from build123d import *


with BuildPart() as f1:
    # F0 (on Front) → F1 (revolve)
    with BuildSketch(Plane.XZ):
        with BuildLine():
            Line((0, 1.241046), (0, 2.482092))
            Line((0, 2.482092), (-22.902938, 2.482092))
            Line((-22.902938, 2.482092), (-22.902938, 0))
            Line((-22.902938, 0), (-24.024541, 0))
            Line((-24.024541, 0), (-30.056966, 73.394649))
            ThreePointArc((-30.056966, 73.394649), (-30.761444, 73.644653), (-30.481581, 72.951496))
            Line((-30.481581, 72.951496), (-24.376155, -1.331323))
            Line((-24.376155, -1.331323), (-22.775946, -1.199799))
            Line((-22.775946, -1.199799), (-21.772536, 1.241046))
            Line((-21.772536, 1.241046), (0, 1.241046))
        make_face()
    revolve(axis=Axis((0, 0, 1.861569), (0, 0, 1)))


solid = f1.part
Input: part model. Units: mm. Frame: model coordinates. A direction names the side the tool comes from. Coordinates: 2 decimals unless noted, no trailing zeros. Loops run counter-clockwise (first coordinate to the right, second up) from the corner with the lowest first, then second, coordinate; pieces in that order, holes last.
(1) Section D-D on z = 56. Return the cut outline in (x, y).
(2) First-contact query: pin 1 Ø12 at (x, z) = (4.5, 17) entering from -Y; pin 2 Ø8 at (x, z) = (24.5, 41) entering from +Y; pin 3 Ø12 at (y, z) = (10, 20.5) entering from +X. Flat tips, straight axial feed; report the tip coordinate or a pass-through.
(3) Pull-direction query (Y, two-part tool) for faces 3 (the face through (5.937, 26.735, 35.29)), 4 (the face through (5.87, 26.44, 37.21)), 5 (the face through (0, 0, 2.482)); classes: released by +Y, released by -Y, zero draft, split by the parting line, or undercut.
(4) Set-up query: faces 1 (the face through (19.5, 12.3, 0)), 2 (the face through (0, 0, 1.241)). Return all of +Z, -Z, +X, -X, +Y, -Y with unobstructed straight access to the full face (end or side cutting, diameter ignored); none if empty.
(5) Section A-A on y = 0. Return the cut outline in (x, z).
(6) Material intervals for probe 1 along Z at (x, y) = (-11.5, -17); probe 2 along X at (y, z) = (-17.5, 7); probe 3 along X at (y, z) = (1.5, 56), sorted ascending.
(7) Section C-C on z = 29. Return the cut outline in (x, y).
Data:
1. outline: circle Ø58.18 at (0, 0); hole circle Ø57.25 at (0, 0)
2. pin 1: stops at y = -26.27
2. pin 2: stops at y = 18.89
2. pin 3: stops at x = 25.98
3. face 3: split by the parting line
3. face 4: undercut
3. face 5: undercut
4. face 1: +Z
4. face 2: -Z
5. outline: (-30.48, 72.95) - (-24.38, -1.33) - (-22.78, -1.2) - (-21.77, 1.24) - (21.77, 1.24) - (22.78, -1.2) - (24.38, -1.33) - (30.48, 72.95) arc R0.41 ccw (long way) to (30.06, 73.39) - (24.02, 0) - (22.9, 0) - (22.9, 2.48) - (-22.9, 2.48) - (-22.9, 0) - (-24.02, 0) - (-30.06, 73.39) arc R0.41 ccw (long way) to start
6. probe 1: z = 1.24 to 2.48
6. probe 2: x = -17.94 to -17.29, 17.29 to 17.94
6. probe 3: x = -29.05 to -28.59, 28.59 to 29.05
7. outline: circle Ø53.74 at (0, 0); hole circle Ø52.82 at (0, 0)
